Build history of the part. All positions in model axes, mm. Face numbers are marked on the shaded views. A direction names the side the tool comes from. Round coordinates to 2 decimals unless told otherwise and drop trailing zeros. Order: outer loops, then holes, each group sorted by start corner. A loop starts at its lowest first (then second) coordinate and runs counter-clockwise, first axis right, second up. Notation, with made-up numbers: M -22.5,15.25 L -18.5,15.25 A20 ccw -18.5,45.25 Z; hole C 65,33.5 d2. An arc over 180 degrees is marked long. One line per item, written item: value. Start each with the question number.
Item 1: Band-saw the part on D-D, the plane x = -3.5. Write the cut outline in (y, z), then the cut area to 3 significant figures.
Item 2: Probe L1, parallel to Y at x = 0, z = 1.75; L2, parallel to Y at x = 0, z = 6.25; L3, parallel to X at y = 0.5, z = 4.5. List the from-to ranges inside material, lowest first.
Item 3: Band-saw the part on A-A, the plane x = 0. Write the cut outline in (y, z).
Item 4: Tool access for the marked faces 4 and 5: list every direction of +Z, -Z, +X, -X, +Y, -Y with a clear straight run to the whole face (end or side of a thin tool).
Item 5: Pin check, flat tips, straight feed: pin 1 (1 mm diameter, centred on y = 13, z = 3.5, fed in from +X); pin 2 (6 mm diameter, centred on x = -8.5, z = 2.5, fed in from -Y); pin 3 (13 mm diameter, centred on x = 0, y = 0, fed in from +Z); pin 4 (4 mm diameter, centred on x = 0, y = -25, fed in from +Z). Stop position of each tip, or through.
Item 6: Band-saw the part on B-B, the plane y = 0. Write the cut outline in (x, z), then the cut area to 3 significant figures.
Item 7: Band-saw the part on C-C, the plane z = 5.75. Write the cut outline in (x, y).
Item 8: Two-plate mould, pull along X, no slides. Class the marked faces 1, 2 and 3: +X half, -X half, draft (parallel to the pull), parting line (faces both ways), or undercut.
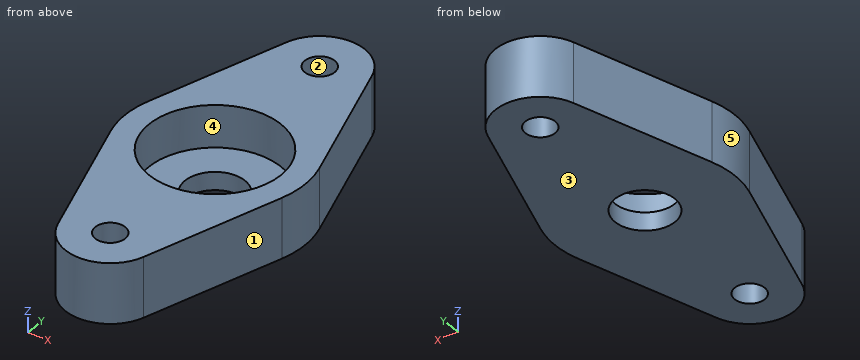
```python
from build123d import *

# Parameters (mm, degrees)
SKETCH_1_R          = 2.5
EXTRUDE_1_DEPTH     = 10
SKETCH_2_R          = 11
CUT_EXTRUDE_1_DEPTH = 7
CUT_EXTRUDE_2_REACH = 5
SKETCH_3_R          = 5


with BuildPart() as part:
    # Эскиз1 → Бобышка-Вытянуть1 (new body)
    with BuildSketch(Plane.XY):
        with BuildLine():
            Line((-14.309088021, 4.5), (-7.154544011, 27.25))
            ThreePointArc((-7.154544011, 27.25), (0, 32.5), (7.154544011, 27.25))
            Line((7.154544011, 27.25), (14.309088021, 4.5))
            ThreePointArc((14.309088021, 4.5), (15, 0), (14.309088021, -4.5))
            Line((14.309088021, -4.5), (7.154544011, -27.25))
            ThreePointArc((7.154544011, -27.25), (0, -32.5), (-7.154544011, -27.25))
            Line((-7.154544011, -27.25), (-14.309088021, -4.5))
            ThreePointArc((-14.309088021, -4.5), (-15, 0), (-14.309088021, 4.5))
        make_face()
        with Locations((0, 25)):
            Circle(SKETCH_1_R, mode=Mode.SUBTRACT)
        with Locations((0, -25)):
            Circle(SKETCH_1_R, mode=Mode.SUBTRACT)
    extrude(amount=EXTRUDE_1_DEPTH)

    # Эскиз2 → Вырез-Вытянуть1 (cut)
    with BuildSketch(Plane.XY.offset(10)):
        Circle(SKETCH_2_R)
    extrude(amount=-CUT_EXTRUDE_1_DEPTH, mode=Mode.SUBTRACT)

    # Эскиз3 → Вырез-Вытянуть2 (cut, up to next)
    with BuildSketch(Plane.XY.offset(3), mode=Mode.PRIVATE) as cut_extrude_2_sk1:
        Circle(SKETCH_3_R)
    cut_extrude_2_tool1 = extrude(cut_extrude_2_sk1.sketch, amount=-CUT_EXTRUDE_2_REACH, mode=Mode.PRIVATE) & part.part
    add(cut_extrude_2_tool1.solids().sort_by_distance((0, 0, 3))[0], mode=Mode.SUBTRACT)


solid = part.part
```
Output:
1. outline: M -31.63,0 L -3.57,0 L -3.57,3 L -10.43,3 L -10.43,10 L -31.63,10 Z; M 3.57,0 L 31.63,0 L 31.63,10 L 10.43,10 L 10.43,3 L 3.57,3 Z
1. area: 465 mm²
2. L1: y = -32.5 to -27.5, -22.5 to -5, 5 to 22.5, 27.5 to 32.5
2. L2: y = -32.5 to -27.5, -22.5 to -11, 11 to 22.5, 27.5 to 32.5
2. L3: x = -14.99 to -10.99, 10.99 to 14.99
3. outline: M -32.5,0 L -27.5,0 L -27.5,10 L -32.5,10 Z; M -22.5,0 L -5,0 L -5,3 L -11,3 L -11,10 L -22.5,10 Z; M 5,0 L 22.5,0 L 22.5,10 L 11,10 L 11,3 L 5,3 Z; M 27.5,0 L 32.5,0 L 32.5,10 L 27.5,10 Z
4. face 4: +Z
4. face 5: +Z, -Z, -X
5. pin 1: stops at x = 11.79
5. pin 2: stops at y = -30.1
5. pin 3: stops at z = 3
5. pin 4: passes through
6. outline: M -15,0 L -5,0 L -5,3 L -11,3 L -11,10 L -15,10 Z; M 5,0 L 15,0 L 15,10 L 11,10 L 11,3 L 5,3 Z
6. area: 116 mm²
7. outline: M -14.31,-4.5 L -7.15,-27.25 A7.5 ccw 7.15,-27.25 L 14.31,-4.5 A15 ccw 14.31,4.5 L 7.15,27.25 A7.5 ccw -7.15,27.25 L -14.31,4.5 A15 ccw Z; hole C 0,0 d22; hole C 0,-25 d5; hole C 0,25 d5
8. face 1: +X half
8. face 2: undercut
8. face 3: draft
